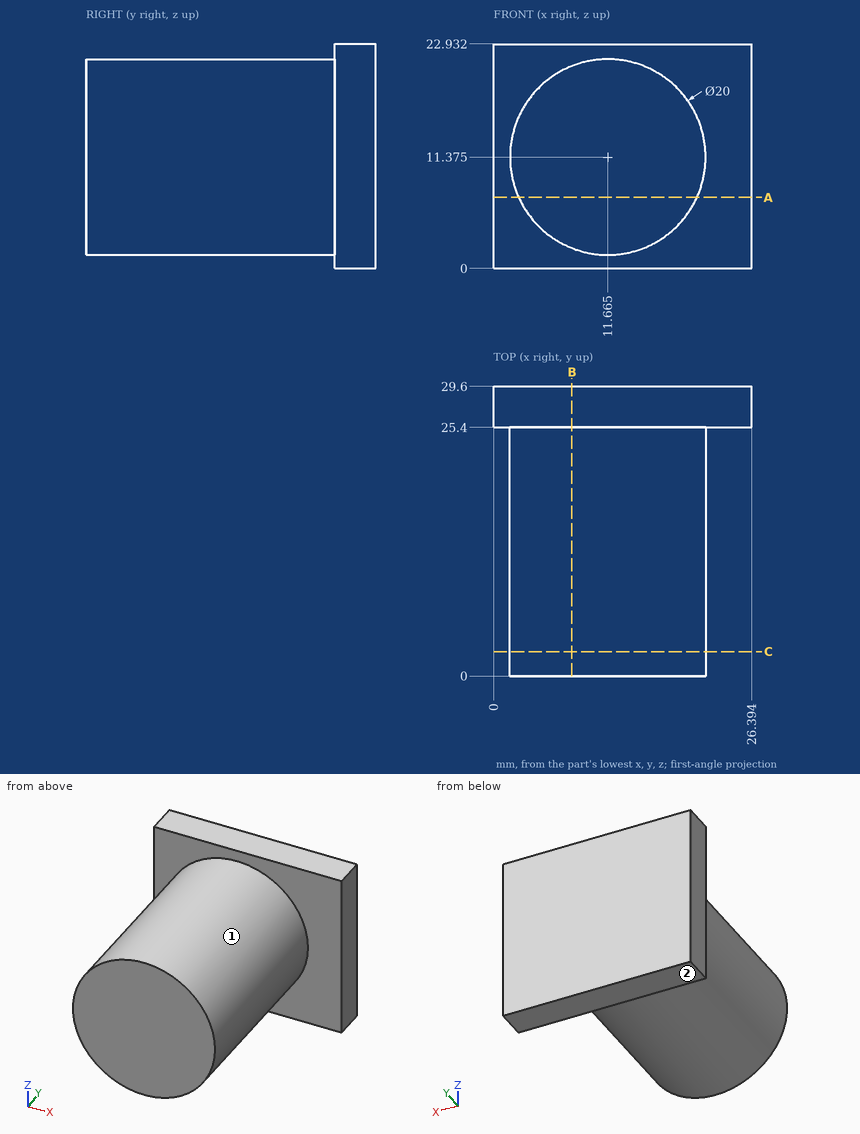
Part print with two shaded views. Sizes in mm from the minimum x, y, z corner. A direction names the side the tool comes from. Round coordinates to 2 decimals unless told otherwise and drop trailing zeros. Order: outer loops, then holes, each group sorted by start corner. A loop starts at its lowest first (then second) coordinate and runs counter-clockwise, first axis right, second up. Notation, with made-up numbers: M 51,7.5 L 73,7.5 A32 ccw 73,39.5 Z; hole C -13,50 d8. An arc over 180 degrees is marked long. Answer in a Markdown table with one row per item. Add a question column.
Q1. Cut at A-A on z = 7.25. Give the cut face in (x, y) (1 decimal).
Q2. Wall check: L1, parallel to Y at x = 22.5, z = 6.75; L2, parallel to X at y = 17, z = 8; L3, parallel to Z at x = 11.25, y = 6. Give the ranges that are in metal, low to high. Write a range as from..to.
Q3. Pin check, flat tips, straight feed: pin 1 (3 mm diameter, centred on x = 13.5, y = 13.5, fed in from -Z); pin 2 (2 mm diameter, centred on y = 5.5, z = 13, fed in from -X); pin 3 (10 mm diameter, centred on y = 17, z = 2.5, fed in from +X). Stop position of each tip, or through.
Q4. Cut at B-B on x = 8. Give the cut face in (y, z), and give its area (3 significant figures).
Q5. 3-axis set-ups, long thin cutter, end or side, ignore diameter. For the marked faces 1 and 2: which of +Z, -Z, +X, -X, +Y, -Y reach the whole face in a straight line?
Q6. Cut at C-C on y = 2.5. Give the cut face in (x, z) (1 decimal).
Established:
| question | item | result |
|---|---|---|
| 1 | outline | M 0,25.4 L 2.6,25.4 L 2.6,0 L 20.8,0 L 20.8,25.4 L 26.4,25.4 L 26.4,29.6 L 0,29.6 Z |
| 2 | L1 | y = 25.4..29.6 |
| 2 | L2 | x = 2.25..21.08 |
| 2 | L3 | z = 1.38..21.37 |
| 3 | pin 1 | stops at z = 1.38 |
| 3 | pin 2 | stops at x = 1.68 |
| 3 | pin 3 | stops at x = 20.88 |
| 4 | outline | M 0,2.07 L 25.4,2.07 L 25.4,0 L 29.6,0 L 29.6,22.93 L 25.4,22.93 L 25.4,20.68 L 0,20.68 Z |
| 4 | area | 569 mm2 |
| 5 | face 1 | -Y |
| 5 | face 2 | -Z, +X, -X, +Y, -Y |
| 6 | outline | C 11.7,11.4 d20 |
